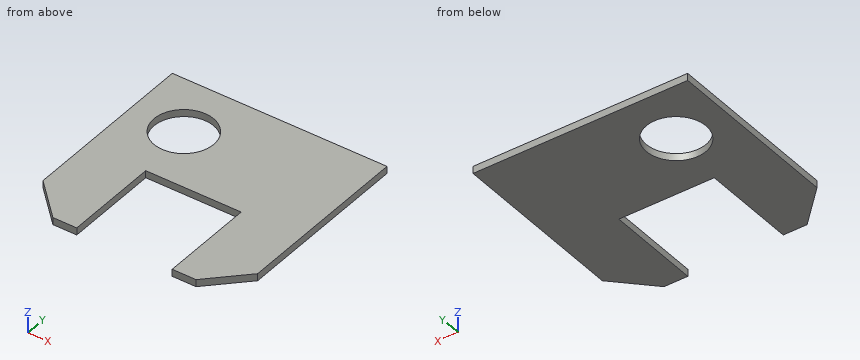
from build123d import *

# Parameters (mm, degrees)
EXTRUSION1_DEPTH        = 3
ESQUISSE2_R             = 12.5
ENL_V_MAT_EXTRU_1_DEPTH = 98.956642072


with BuildPart() as part:
    # Esquisse1 → Extrusion1 (new body)
    with BuildSketch(Plane.XY):
        Polygon((3.720449438, -58.220224719), (-11.279550562, -43.220224719), (-11.279550562, 31.779775281), (33.720449438, 31.779775281), (33.720449438, -18.220224719), (13.720449438, -18.220224719), (13.720449438, -58.220224719), align=None)
    extrusion1 = extrude(amount=EXTRUSION1_DEPTH)

    # Symétrie1: Extrusion1 across plane
    add(extrusion1.mirror(Plane(origin=(33.720449438, 31.779775281, 3), x_dir=(0, 0, 1), z_dir=(-1, 0, 0))))

    # Esquisse2 → Enlèv. mat.-Extru.1 (cut, through all)
    with BuildSketch(Plane.XY.offset(3)):
        with Locations((11.220449438, 7.325247065)):
            Circle(ESQUISSE2_R)
    extrude(amount=-ENL_V_MAT_EXTRU_1_DEPTH, mode=Mode.SUBTRACT)


solid = part.part
Could you check a few things on this model? Use its own coordinates, in mm. Coordinates: 2 decimals unless noted, no trailing zeros. Write each loop counter-clockwise with the first axis right and the second up, starting at its lowest first coordinate (ties: lowest second). Pieces come first, ordered by that corner, then holes. Notation, with made-up numbers: (-2.75, -38) - (22.25, -38) arc R27 ccw to (22.25, -6) - close; hole circle Ø4 at (-23.5, 81). An arc over 180 degrees is marked (long way). Put each result on its own line as item: value. Start each with the question number.
Q1. I want a section at A-A on y = -25. Write out the boundary of the cut face in (x, z).
Q2. I want a section at C-C on x = 12.5. Write out the boundary of the cut face in (y, z).
Q3. I want a section at D-D on x = 46.5. Write out the boundary of the cut face in (y, z), plus the area to 3 significant figures.
Q4. I want a section at B-B on z = 0.5. Write out the boundary of the cut face in (x, y), plus the area to 3 significant figures.
Q5. Please list where these lines run through material, in increasing order: L1, parallel to X at y = -21, z = 0.6; L2, parallel to X at y = -53.5, z = 1.35; L3, parallel to Y at x = 3, z = 0.1.
Q6. I'm going to push a flat-ended pin straight in: P1, Ø0.9, axis at x = 30.5, z = 1.5, coming from the -Y side. Where does the tip first touch, or does it pass through?
Checks:
1. outline: (-11.28, 0) - (13.72, 0) - (13.72, 3) - (-11.28, 3) - close; (53.72, 0) - (78.72, 0) - (78.72, 3) - (53.72, 3) - close
2. outline: (-58.22, 0) - (-5.11, 0) - (-5.11, 3) - (-58.22, 3) - close; (19.76, 0) - (31.78, 0) - (31.78, 3) - (19.76, 3) - close
3. outline: (-18.22, 0) - (31.78, 0) - (31.78, 3) - (-18.22, 3) - close
3. area: 150 mm²
4. outline: (-11.28, -43.22) - (3.72, -58.22) - (13.72, -58.22) - (13.72, -18.22) - (53.72, -18.22) - (53.72, -58.22) - (63.72, -58.22) - (78.72, -43.22) - (78.72, 31.78) - (-11.28, 31.78) - close; hole circle Ø25 at (11.22, 7.33)
4. area: 5,780 mm²
5. L1: -11.28 to 13.72, 53.72 to 78.72
5. L2: -1 to 13.72, 53.72 to 68.44
5. L3: -57.5 to -2.09, 16.74 to 31.78
6. P1: y = -18.22
